Check sheet for the modelled part. Datum: model origin and axes. Units: mm. Face numbers are marked on the shaded views. A direction names the side the tool comes from. Give positions to 0.01 mm unless a question says otherwise; leave off trailing zeros. Write each loop counter-clockwise with the first axis right and the second up, starting at its lowest first coordinate (ties: lowest second). Pieces come first, ordered by that corner, then holes. Notation, with made-up numbers: M 24,-5.5 L 69,-5.5 A18 ccw 69,18.5 Z; hole C 67.25,32 d5. An arc over 180 degrees is marked long. One line per item, written item: value. Start each with the question number.
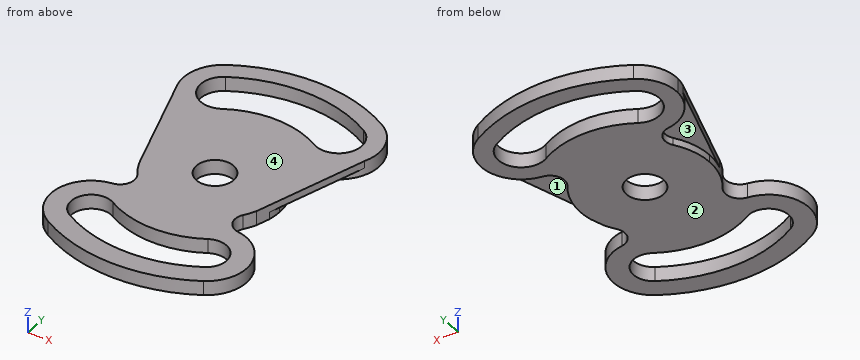
Autodesk Inventor part; units mm, degrees
ref_plane "YZ Plane" through (0, 0, 0) normal (1, 0, 0) x (0, 1, 0)
ref_plane "XZ Plane" through (0, 0, 0) normal (0, 1, 0) x (-1, 0, 0)
ref_plane "XY Plane" through (0, 0, 0) normal (0, 0, 1) x (1, 0, 0)
sketch "Эскиз1" plane through (0, 0, 0) normal (0, 0, 1) x (1, 0, 0)
  circle A0 centre (120.236, 134.1079) radius 13
  arc A1 (165.236, 134.1079) -> (157.0596, 159.9734) centre (120.236, 134.1079) ccw
  arc A2 (168.236, 217.2464) -> (72.236, 217.2464) centre (120.236, 134.1079) ccw
  arc A3 (152.236, 189.5336) -> (88.236, 189.5336) centre (120.236, 134.1079) ccw
  arc A4 (152.236, 189.5336) -> (168.236, 217.2464) centre (160.236, 203.39) ccw
  arc A5 (72.236, 217.2464) -> (88.236, 189.5336) centre (80.236, 203.39) ccw
  arc A6 (174.236, 227.6387) -> (66.236, 227.6387) centre (120.236, 134.1079) ccw
  arc A7 (66.236, 227.6387) -> (52.275, 201.9114) centre (80.236, 203.39) ccw
  line L0 (68.236, 134.1079) -> (172.236, 134.1079)
  arc A8 (75.236, 134.1079) -> (83.4123, 108.2425) centre (120.236, 134.1079) ccw
  arc A9 (52.275, 201.9114) -> (76.5468, 175.6341) centre (80.236, 203.39) ccw
  line L1 (120.236, 242.1079) -> (120.236, 26.1079)
  arc A10 (73.236, 52.7015) -> (167.236, 52.7015) centre (120.236, 134.1079) ccw
  arc A11 (87.236, 76.9503) -> (153.236, 76.9503) centre (120.236, 134.1079) ccw
  arc A12 (87.236, 76.9503) -> (73.236, 52.7015) centre (80.236, 64.8259) ccw
  arc A13 (167.236, 52.7015) -> (153.236, 76.9503) centre (160.236, 64.8259) ccw
  arc A14 (66.236, 40.5772) -> (174.236, 40.5772) centre (120.236, 134.1079) ccw
  arc A15 (174.236, 40.5772) -> (163.9251, 92.5818) centre (160.236, 64.8259) ccw
  arc A16 (76.5468, 92.5818) -> (83.4123, 108.2425) centre (75.2293, 102.4946) ccw
  arc A17 (157.0596, 108.2425) -> (163.9251, 92.5818) centre (165.2426, 102.4946) ccw
  arc A18 (157.0596, 108.2425) -> (165.236, 134.1079) centre (120.236, 134.1079) ccw
  arc A19 (76.5468, 92.5818) -> (66.236, 40.5772) centre (80.236, 64.8259) ccw
  arc A20 (83.4123, 159.9734) -> (76.5468, 175.6341) centre (75.2293, 165.7212) ccw
  arc A21 (83.4123, 159.9734) -> (75.236, 134.1079) centre (120.236, 134.1079) ccw
  arc A22 (163.9251, 175.6341) -> (157.0596, 159.9734) centre (165.2426, 165.7212) ccw
  arc A23 (163.9251, 175.6341) -> (174.236, 227.6387) centre (160.236, 203.39) ccw
  line L2 (161.3771, 115.876) -> (185.8349, 192.0456)
  arc A24 (58.8114, 82.8534) -> (181.6605, 82.8534) centre (120.236, 134.1079) ccw
  arc A25 (181.6605, 185.3625) -> (58.8114, 185.3625) centre (120.236, 134.1079) ccw
  line L3 (120.236, 134.1079) -> (66.236, 40.5772)
  line L4 (120.236, 134.1079) -> (174.236, 40.5772)
  line L5 (120.236, 134.1079) -> (66.236, 227.6387)
  line L6 (120.236, 134.1079) -> (174.236, 227.6387)
  line L7 (53.5661, 194.8626) -> (77.3736, 120.4032)
  point P0 (164.3006, 124.9806)
  point P1 (165.236, 134.1079)
  point P2 (167.2313, 134.1079)
  dimension "d122" = 10
  dimension "d123" = 28
  dimension "d124" = 16
  dimension "d125" = 14
  dimension "d126" = 108
  dimension "d127" = 45
  dimension "d128" = 26
  dimension "d130" = 12.198
  dimension "d131" = 47.802
  dimension "d133" = 0
  dimension "d134" = 4.765
  dimension "d135" = 1.8998
  dimension "d139" = 94.2555
  dimension "d153" = 44.7453
  dimension "d154" = 55.683
  dimension "d155" = 0
  dimension "d156" = 55.683
  dimension "d157" = 0
  dimension "d158" = 81.3984
  dimension "d159" = 1.8998
  dimension "d160" = 77.9423
  dimension "d161" = 0
  dimension "d162" = 85.4495
  dimension "d163" = 89.4905
  dimension "d164" = 0
  dimension "d165" = 89.4905
extrude "Выдавливание3" add sketch "Эскиз1" against normal blind 5 contours L0 A18 L2 A17 A15 A24 A13 L4 A0 | A0 L6 A4 A25 A23 A22 A1 L0 | A0 L1 A3 L6 | L4 A11 L1 A0 | A1 A22 A23 L2 L0 | L0 L2 A18 | A0 L5 A3 L1 | L1 A11 L3 A0 | L0 A21 A20 A9 A25 A5 L5 A0 | A0 L3 A12 A24 A19 A16 A8 L0 | A4 L6 A23 A25 | A24 A15 L4 A13 | A8 L7 L0 | L0 L7 A9 A20 A21 | A2 L1 A6 L6 | L4 A14 L1 A10 | A12 L3 A19 A24 | A25 A9 A7 L5 A5 | A2 L5 A6 L1 | L1 A14 L3 A10
extrude "Выдавливание4" add sketch "Эскиз1" against normal blind 10 contours L0 A18 L2 A17 A15 A24 A13 L4 A0 | A0 L6 A4 A25 A23 A22 A1 L0 | A0 L1 A3 L6 | L4 A11 L1 A0 | A0 L5 A3 L1 | L1 A11 L3 A0 | L0 A21 A20 A9 A25 A5 L5 A0 | A0 L3 A12 A24 A19 A16 A8 L0 | A4 L6 A23 A25 | A24 A15 L4 A13 | A2 L1 A6 L6 | L4 A14 L1 A10 | A12 L3 A19 A24 | A25 A9 A7 L5 A5 | A2 L5 A6 L1 | L1 A14 L3 A10
properties part number "3.2"
1) Cross-section at B-B (z = -1.5). Record the boundary of the cut face in (x, y) (1 decimal).
2) Draft check along Y on the marked faces 1 and 2. Enter one of: released by +Y, released by -Y, zero draft, split by the parting line, or undercut.
3) Cross-section at D-D (y = 47.5). Record the boundary of the cut face in (x, z), plus the area to 3 significant figures.
4) Material ranges on L1, parallel to Y at x = 144.5, z = -2.25; L2, parallel to Y at x = 144, z = -4.75; L3, parallel to Y at x = 129.5, z = -3.75, recorded low to high. Write a range as from..to.
5) Cross-section at A-A (y = 129). Record the boundary of the cut face in (x, z), plus the area to 3 significant figures.
6) Cross-section at C-C (x = 119). Record the boundary of the cut face in (y, z).
7) Tool access check on the marked faces 3 and 4. Record the directions out of +Z, -Z, +X, -X, +Y, -Y that give a thin tool (end or side, any length) a straight path to the whole face; none if there is none.
8) Gauge pin test, flat ends, axial feed: pin 1 (1.5 mm diameter, centred on x = 83.5, z = -5, fed in from -Y); pin 2 (2 mm diameter, centred on x = 104.5, z = -5, fed in from -Y); pin 3 (1 mm diameter, centred on x = 172.5, z = -6.5, fed in from +Y). Record the tip position at first contact, or that the pin passes through.
Data:
1. outline: M 52.3,201.9 A28 ccw 53.6,194.9 L 77.4,120.4 A45 ccw 83.4,108.2 A10 cw 76.5,92.6 A28 ccw 66.2,40.6 A108 ccw 174.2,40.6 A28 ccw 163.9,92.6 A10 cw 157.1,108.2 A45 ccw 161.4,115.9 L 185.8,192 A28 ccw 174.2,227.6 A108 ccw 66.2,227.6 A28 ccw Z; hole M 72.2,217.2 A16 ccw 88.2,189.5 A64 cw 152.2,189.5 A16 ccw 168.2,217.2 A96 ccw Z; hole M 73.2,52.7 A94 ccw 167.2,52.7 A14 ccw 153.2,77 A66 cw 87.2,77 A14 ccw Z; hole C 120.2,134.1 d26
2. face 1: undercut
2. face 2: zero draft
3. outline: M 58.24,-10 L 83.7,-10 L 83.7,0 L 58.24,0 Z; M 156.77,-10 L 182.23,-10 L 182.23,0 L 156.77,0 Z
3. area: 509 mm2
4. L1: y = 28.87..43.29, 72.73..193.33, 226.99..239.35
4. L2: y = 28.75..43.16, 72.53..193.53, 227.12..239.46
4. L3: y = 26.51..40.57, 68.76..124.99, 143.23..197.43, 229.66..241.71
5. outline: M 74.62,-5 L 75.53,-5 L 75.53,-10 L 108.28,-10 L 108.28,0 L 74.62,0 Z; M 132.19,-10 L 164.95,-10 L 164.95,-5 L 165.59,-5 L 165.59,0 L 132.19,0 Z
5. area: 663 mm2
6. outline: M 26.12,-10 L 40.12,-10 L 40.12,0 L 26.12,0 Z; M 68.12,-10 L 121.17,-10 L 121.17,0 L 68.12,0 Z; M 147.05,-10 L 198.1,-10 L 198.1,0 L 147.05,0 Z; M 230.1,-10 L 242.1,-10 L 242.1,0 L 230.1,0 Z
7. face 3: -Z, -X
7. face 4: +Z, +X, -X, +Y, -Y
8. pin 1: stops at y = 32.28
8. pin 2: stops at y = 27.12
8. pin 3: stops at y = 228.89
